Work out the finished part from the listing and answer in its coordinate system (mm). Round coordinates to 2 decimals unless told otherwise and drop trailing zeros. Loops run counter-clockwise (first coordinate to the right, second up) from the corner with the lowest first, then second, coordinate; pieces in that order, holes last. Notation, with made-up numbers: (77, 59.25) - (102, 59.25) arc R17 cw to (102, 63.25) - close; hole circle Ø6 at (76.5, 11.5). An arc over 180 degrees is marked (long way). Answer as CSV lines item,"result". Start each with the question number.
```python
from build123d import *

# Parameters (mm, degrees)
F1_DEPTH = 38.1
F3_DEPTH = 101.6
F5_DEPTH = 127


with BuildPart() as f1:
    # F0 (on Front) → F1 (new body)
    with BuildSketch(Plane.XZ):
        with BuildLine():
            Line((27.7732536197, -17.7548748881), (27.7732536197, 20.3451251119))
            ThreePointArc((27.7732536197, 20.3451251119), (23.3150850981, 19.0968449339), (18.8569165766, 20.3451251119))
            Line((18.8569165766, 20.3451251119), (-24.5568101805, 46.7248205056))
            Line((-24.5568101805, 46.7248205056), (-24.5568101805, -40.3753659966))
            Line((-24.5568101805, -40.3753659966), (20.0085155666, -17.7548748881))
            ThreePointArc((20.0085155666, -17.7548748881), (23.8908845931, -16.8259725337), (27.7732536197, -17.7548748881))
        make_face()
    extrude(amount=F1_DEPTH)

    # F2 (on face) → F3 (cut)
    with BuildSketch(Plane(origin=(11.2647537366, 0, -22.1930380433), x_dir=(0.8917070033, 0, 0.4526131022), z_dir=(0.4526131022, 0, -0.8917070033))):
        Polygon((-40.1718992738, 0), (9.8056444527, 0), (-40.1718992738, 17.5163969398), align=None)
        Polygon((-40.1718992738, 19.8567565531), (9.8056444527, 38.1), (-40.1718992738, 38.1), align=None)
    extrude(amount=-F3_DEPTH, mode=Mode.SUBTRACT)

    # F4 (on face) → F5 (cut)
    with BuildSketch(Plane(origin=(14.113699436, 0, 23.2272693714), x_dir=(0.8546009204, 0, -0.5192853424), z_dir=(0.5192853424, 0, 0.8546009204))):
        Polygon((-25.222287783, -38.1), (5.5502130028, -38.1), (-45.2497869972, -22.2575453606), (-45.2497869972, -34.247172677), align=None)
        Polygon((-45.2497869972, -14.9671534034), (5.5502130028, 0), (-25.222287783, 0), (-45.2497869972, -3.6993231454), align=None)
    extrude(amount=-F5_DEPTH, mode=Mode.SUBTRACT)


solid = f1.part
```
Item 1: Flat-ended cylindrical pins translate along their axes: pin 1 Ø2 at (x, z) = (-7.5, -0.5) entering from -Y; pin 2 Ø2 at (x, y) = (18, -9) entering from -Z; pin 3 Ø6 at (x, y) = (12.5, -10.5) entering from -Z. Find the tip coordinate at first contact, or state that the pin passes through.
Item 2: Section C-C, the plane x = 2 is taken. Give the vertices of the cut face in (y, z), and give its area (3 significant figures).
Item 3: Find the intervals of material crossed by L1, parallel to Z at x = 16.5, y = -22; L2, parallel to Y at x = -13, z = 35.5; L3, parallel to X at y = -14, z = 40, in increasing order.
Item 4: Section B-B, the plane z = 17 is taken. Give the vertices of the cut face in (x, y).
Item 5: Section D-D, the plane y = -5 is taken. Give the vertices of the cut face in (x, z).
Item 6: Determine the mould class of faces 1 (the face through (-5.41, -30.88, -11.39)), 2 (the face through (23.381, -18.783, 19.097)), 3 (the face through (27.773, -19, 1)) for opening direction X: pulls with the +X half, pulls with the -X half, needs draft (parallel to the pull), parting line crosses it, or undercut.
Item 7: Section A-A, the plane y = -31 is taken. Give the vertices of the cut face in (x, z), and give its area (3 significant figures).
Answer:
1,pin 1,"stops at y = -32.36"
1,pin 2,"stops at z = -19.28"
1,pin 3,"stops at z = -23.09"
2,outline,"(-36.05, 5.29) - (-30.73, -26.9) - (-7.08, -26.9) - (-1.96, 5.39) - (-5.81, 30.59) - (-31.95, 30.59) - close"
2,area,"1,690 mm²"
3,L1,"z = -19.54 to 21.78"
3,L2,"y = -27.16 to -10.34"
3,L3,"x = -24.56 to -13.49"
4,outline,"(-24.56, -27.07) - (16.82, -38.1) - (27.77, -38.1) - (27.77, 0) - (16.82, 0) - (-24.56, -10.42) - close"
5,outline,"(-8.81, 7.5) - (7.29, -24.21) - (20.01, -17.75) arc R8.58 cw to (27.77, -17.75) - (27.77, 20.35) arc R8.59 cw to (18.86, 20.35) - (4.35, 29.16) - close"
6,face 1,"pulls with the -X half"
6,face 2,"undercut"
6,face 3,"pulls with the +X half"
7,outline,"(-15.06, 8.37) - (2.66, -26.56) - (20.01, -17.75) arc R8.58 cw to (27.77, -17.75) - (27.77, 20.35) arc R8.59 cw to (18.86, 20.35) - (-0.6, 32.17) - close"
7,area,"1,660 mm²"
